Read the model definition and answer for the solid it produces. Units are mm, in the model's axes. A direction names the side the tool comes from. Give positions to 0.01 mm unless a question says otherwise; leave off trailing zeros. Order: outer loops, then holes, each group sorted by start corner. A loop starts at its lowest first (then second) coordinate and runs counter-clockwise, first axis right, second up. Notation, with made-up numbers: (33, -21) - (43, -21) arc R11 ccw to (43, -14) - close; hole circle Ø3 at (31, 68.5). An arc over 180 degrees is marked (long way). Use a Markdown table: item, result. Add a question column.
1. A cutting plane is placed at C-C on y = 0. Determine the outline of the cut face in (x, z).
2. Consider L1, parallel to X at y = -1.5, z = 5; L2, parallel to Z at x = 2, y = 4; L3, parallel to X at y = 3, z = 3. Determine where each line is inside the solid, lowest interval first.
3. A cutting plane is placed at B-B on x = 0. Determine the outline of the cut face in (y, z).
4. Which of the six approach directions +Z, -Z, +X, -X, +Y, -Y give full straight-line access (tool end or side, diameter ignored) to faces 4 (the cylindrical face through (0, -8, 3)), 5 (the flat face through (-6.75, 0, 3)), 6 (the cylindrical face through (-0.07, 5.75, 3.3))?
5. A cutting plane is placed at D-D on z = -1.5. Determine the outline of the cut face in (x, y).
6. For a pull along X with two mould halves and no side action, classify faces 1 (the cylindrical face through (0, 8, 3)), 2 (the flat face through (6.75, 0, 3)), 3 (the flat face through (0, 0, 0)) as released by +X, released by -X, zero draft, split by the parting line, or undercut.
7. Flat-ended cylindrical pins translate along their axes: P1, Ø2, axis at x = -5, z = -1.5, coming from the -Y side; P2, Ø1, axis at x = 1, z = -0.5, coming from the +Y side; P3, Ø3, axis at y = 0.5, z = 2.5, coming from the -X side. Find the tip coordinate at first contact, or state that the pin passes through.
```python
from build123d import *

# Parameters (mm, degrees)
F0_R     = 11.5
F1_DEPTH = 3
F2_R     = 1.2
F3_DEPTH = 6.7


with BuildPart() as f1:
    # F0 (on Top) → F1 (new body)
    with BuildSketch(Plane.XY):
        Circle(F0_R)
        with BuildLine():
            ThreePointArc((-6.75, 1.25), (0, 8), (6.75, 1.25))
            Line((6.75, 1.25), (6.75, -1.25))
            ThreePointArc((6.75, -1.25), (0, -8), (-6.75, -1.25))
            Line((-6.75, -1.25), (-6.75, 1.25))
        make_face(mode=Mode.SUBTRACT)
        with BuildLine():
            ThreePointArc((4.5, 4.20141), (5.815353, 2.87082), (6.75, 1.25))
            ThreePointArc((6.75, 1.25), (0, 8), (-6.75, 1.25))
            ThreePointArc((-6.75, 1.25), (-5.815353, 2.87082), (-4.5, 4.20141))
            ThreePointArc((-4.5, 4.20141), (0, 5.75), (4.5, 4.20141))
        make_face()
        with BuildLine():
            ThreePointArc((-4.5, 4.20141), (-5.815353, 2.87082), (-6.75, 1.25))
            Line((-6.75, 1.25), (-6.75, -1.25))
            ThreePointArc((-6.75, -1.25), (-5.815353, -2.87082), (-4.5, -4.20141))
            Line((-4.5, -4.20141), (-4.5, 4.20141))
        make_face()
        with BuildLine():
            Line((4.5, -4.20141), (4.5, 4.20141))
            ThreePointArc((4.5, 4.20141), (0, 5.75), (-4.5, 4.20141))
            Line((-4.5, 4.20141), (-4.5, -4.20141))
            ThreePointArc((-4.5, -4.20141), (0, -5.75), (4.5, -4.20141))
        make_face()
        with BuildLine():
            ThreePointArc((-6.75, -1.25), (0, -8), (6.75, -1.25))
            ThreePointArc((6.75, -1.25), (5.815353, -2.87082), (4.5, -4.20141))
            ThreePointArc((4.5, -4.20141), (0, -5.75), (-4.5, -4.20141))
            ThreePointArc((-4.5, -4.20141), (-5.815353, -2.87082), (-6.75, -1.25))
        make_face()
        with BuildLine():
            Line((6.75, -1.25), (6.75, 1.25))
            ThreePointArc((6.75, 1.25), (5.815353, 2.87082), (4.5, 4.20141))
            Line((4.5, 4.20141), (4.5, -4.20141))
            ThreePointArc((4.5, -4.20141), (5.815353, -2.87082), (6.75, -1.25))
        make_face()
    extrude(amount=-F1_DEPTH)

    # F2
    f2_edges = [f1.edges().sort_by_distance(p)[0] for p in [
        (-11.5, 0, -3),
    ]]
    fillet(f2_edges, radius=F2_R)

    # F0 (on Top) → F3 (join)
    with BuildSketch(Plane.XY):
        with BuildLine():
            ThreePointArc((-4.5, 4.20141), (-5.815353, 2.87082), (-6.75, 1.25))
            Line((-6.75, 1.25), (-6.75, -1.25))
            ThreePointArc((-6.75, -1.25), (-5.815353, -2.87082), (-4.5, -4.20141))
            Line((-4.5, -4.20141), (-4.5, 4.20141))
        make_face()
        with BuildLine():
            ThreePointArc((4.5, 4.20141), (5.815353, 2.87082), (6.75, 1.25))
            ThreePointArc((6.75, 1.25), (0, 8), (-6.75, 1.25))
            ThreePointArc((-6.75, 1.25), (-5.815353, 2.87082), (-4.5, 4.20141))
            ThreePointArc((-4.5, 4.20141), (0, 5.75), (4.5, 4.20141))
        make_face()
        with BuildLine():
            Line((6.75, -1.25), (6.75, 1.25))
            ThreePointArc((6.75, 1.25), (5.815353, 2.87082), (4.5, 4.20141))
            Line((4.5, 4.20141), (4.5, -4.20141))
            ThreePointArc((4.5, -4.20141), (5.815353, -2.87082), (6.75, -1.25))
        make_face()
        with BuildLine():
            ThreePointArc((-6.75, -1.25), (0, -8), (6.75, -1.25))
            ThreePointArc((6.75, -1.25), (5.815353, -2.87082), (4.5, -4.20141))
            ThreePointArc((4.5, -4.20141), (0, -5.75), (-4.5, -4.20141))
            ThreePointArc((-4.5, -4.20141), (-5.815353, -2.87082), (-6.75, -1.25))
        make_face()
    extrude(amount=F3_DEPTH)


solid = f1.part
```
Output values:
| question | item | result |
|---|---|---|
| 1 | outline | (-11.5, -1.8) arc R1.2 ccw to (-10.3, -3) - (10.3, -3) arc R1.2 ccw to (11.5, -1.8) - (11.5, 0) - (6.75, 0) - (6.75, 6.7) - (4.5, 6.7) - (4.5, 0) - (-4.5, 0) - (-4.5, 6.7) - (-6.75, 6.7) - (-6.75, 0) - (-11.5, 0) - close |
| 2 | L1 | -6.75 to -4.5, 4.5 to 6.75 |
| 2 | L2 | -3 to 0 |
| 2 | L3 | -6.52 to -4.5, 4.5 to 6.52 |
| 3 | outline | (-11.5, -1.8) arc R1.2 ccw to (-10.3, -3) - (10.3, -3) arc R1.2 ccw to (11.5, -1.8) - (11.5, 0) - (8, 0) - (8, 6.7) - (5.75, 6.7) - (5.75, 0) - (-5.75, 0) - (-5.75, 6.7) - (-8, 6.7) - (-8, 0) - (-11.5, 0) - close |
| 4 | face 4 | +Z, -Y |
| 4 | face 5 | +Z, -X, +Y, -Y |
| 4 | face 6 | +Z |
| 5 | outline | circle Ø23 at (0, 0) |
| 6 | face 1 | split by the parting line |
| 6 | face 2 | released by +X |
| 6 | face 3 | undercut |
| 7 | P1 | y = -10.78 |
| 7 | P2 | y = 11.49 |
| 7 | P3 | x = -6.75 |
